Read the model definition and answer for the solid it produces. Units are mm, in the model's axes. Give positions to 0.01 mm unless a question says otherwise; leave off trailing zeros. Order: outer loops, then holes, each group sorted by start corner. A loop starts at its lowest first (then second) coordinate and runs counter-clockwise, first axis right, second up. Notation, with made-up numbers: (-14, 37) - (27, 37) arc R25 ccw to (27, 50) - close; hole circle Ø5 at (71.25, 50). An arc over 180 degrees is marked (long way). Write item = value, one per line.
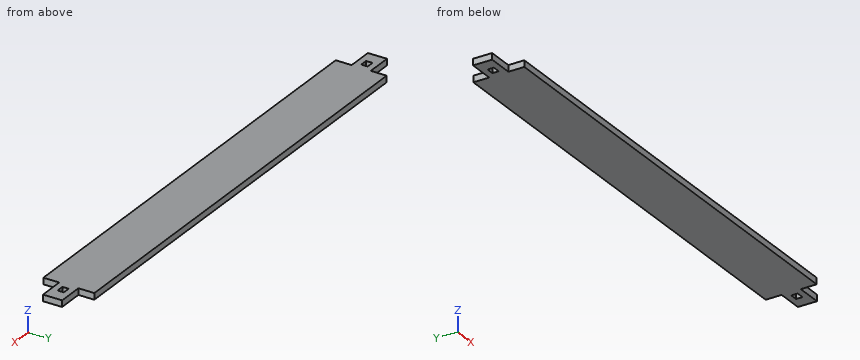
```python
from build123d import *

# Parameters (mm, degrees)
SKETCH1_W           = 457.2
SKETCH1_H           = 50.8
BOSS_EXTRUDE1_DEPTH = 6.35
SKETCH2_W           = 50.8
SKETCH2_H           = 19.05
BOSS_EXTRUDE2_DEPTH = 6.35
SKETCH3_W           = 7.62
SKETCH3_H           = 6.35
CUT_EXTRUDE1_DEPTH  = 7.35


with BuildPart() as part:
    # Sketch1 → Boss-Extrude1 (new body)
    with BuildSketch(Plane.XY):
        Rectangle(SKETCH1_W, SKETCH1_H)
    extrude(amount=BOSS_EXTRUDE1_DEPTH)

    # Sketch2 → Boss-Extrude2 (add)
    with BuildSketch(Plane.XY.offset(6.35)):
        with Locations((-228.6, 0)):
            Rectangle(SKETCH2_W, SKETCH2_H)
    boss_extrude2 = extrude(amount=-BOSS_EXTRUDE2_DEPTH)

    # Sketch3 → Cut-Extrude1 (cut, through all)
    with BuildSketch(Plane.XY.offset(6.35)):
        with Locations((-237.49, 0)):
            Rectangle(SKETCH3_W, SKETCH3_H)
    cut_extrude1 = extrude(amount=-CUT_EXTRUDE1_DEPTH, mode=Mode.SUBTRACT)

    # Mirror1: Boss-Extrude2, Cut-Extrude1 across plane
    add(boss_extrude2.mirror(Plane(origin=(0, 0, 0), x_dir=(0, 0, 1), z_dir=(1, 0, 0))))
    add(cut_extrude1.mirror(Plane(origin=(0, 0, 0), x_dir=(0, 0, 1), z_dir=(1, 0, 0))), mode=Mode.SUBTRACT)


solid = part.part
```
1. Section B-B (y = 17) is taken. Determine the outline of the cut face in (x, z), and give its area (3 significant figures).
Recorded:
outline = (-228.6, 0) - (228.6, 0) - (228.6, 6.35) - (-228.6, 6.35) - close
area = 2,900 mm^2
2. Flat-ended cylindrical pins translate along their axes: pin 1 (2 mm diameter, centred on y = 13.5, z = 4, fed in from -X); pin 2 (1.9 mm diameter, centred on x = 244, z = 2.5, fed in from -Y) (3 decimals); pin 3 (1.9 mm diameter, centred on y = -15, z = 1.5, fed in from +X). Find the tip coordinate at first contact, or state that the pin passes through.
Recorded:
pin_1 = -228.6
pin_2 = -9.525
pin_3 = 228.6
3. Section A-A (z = 5) is taken. Determine the outline of the cut face in (x, y) (3 decimals).
Recorded:
outline = (-254, -9.525) - (-228.6, -9.525) - (-228.6, -25.4) - (228.6, -25.4) - (228.6, -9.525) - (254, -9.525) - (254, 9.525) - (228.6, 9.525) - (228.6, 25.4) - (-228.6, 25.4) - (-228.6, 9.525) - (-254, 9.525) - close; hole (-241.3, -3.175) - (-233.68, -3.175) - (-233.68, 3.175) - (-241.3, 3.175) - close; hole (233.68, -3.175) - (241.3, -3.175) - (241.3, 3.175) - (233.68, 3.175) - close
4. Straight lines are drawn through the part: L1, parallel to X at y = 1, z = 4.5; L2, parallel to X at y = -23, z = 6. For each, find the intervals that lie inside material, in ascending order. Write a range as [from, to].
Recorded:
L1 = [-254, -241.3], [-233.68, 233.68], [241.3, 254]
L2 = [-228.6, 228.6]
